Geometry check sheet. Reference: the model listing, model coordinates, mm. A direction names the side the tool comes from. Give positions to 0.01 mm unless a question says otherwise; leave off trailing zeros. Loops run counter-clockwise (first coordinate to the right, second up) from the corner with the lowest first, then second, coordinate; pieces in that order, holes last.
1. Cross-section at D-D, the plane z = 15. Record the cut outline in (x, y) (3 decimals), plus the area to 3 significant figures.
2. Release check for a two-part mould opening along Z. For faces 3 (the flat face through (29, 0, -10)), 4 (the cylindrical face through (26.91, -10.46, 0.07)), 5 (the cylindrical face through (30.15, -5.63, -12.5)) record: +Z half, -Z half, draft (parallel to the pull), parting line (faces both ways), or undercut.
3. Material ranges on L1, parallel to Z at x = 0, y = -5.75; L2, parallel to Y at x = -23, z = 17.5 (3 decimals); L3, parallel to X at y = -7.5, z = -22.5, recorded low to high.
4. Cross-section at C-C, the plane x = 0. Record the cut outline in (y, z) (3 decimals).
5. Cross-section at B-B, the plane z = 0. Record the cut outline in (x, y) (3 decimals), plus the area to 3 significant figures.
6. Tool access check on faces 1 (the cylindrical face through (-23.89, -10.46, 0.07)), 2 (the flat face through (0, -9.525, 0)). Record the directions out of +Z, -Z, +X, -X, +Y, -Y that give a thin tool (end or side, any length) a straight path to the whole face; none if there is none.
7. Cross-section at A-A, the plane x = 25.4. Record the cut outline in (y, z) (3 decimals).
8. Go/stop test with flat-tipped pins: pin 1 Ø4 at (x, z) = (-7.5, 2) entering from +Y (3 decimals); pin 2 Ø4 at (x, y) = (6.5, -9) entering from -Z; pin 3 Ø4 at (x, y) = (-24.5, -7.5) entering from +Z. Record where each tip stops, or that it passes through.
from build123d import *

# Parameters (mm, degrees)
F0_R     = 32.639
F1_DEPTH = 11.43
F2_R     = 30.353
F3_DEPTH = 9.525
F4_R     = 1.5113
F5_DEPTH = 1.905


with BuildPart() as f1:
    # F0 (on Front) → F1 (new body)
    with BuildSketch(Plane.XZ):
        Circle(F0_R)
    extrude(amount=F1_DEPTH)

    # F2 (on face) → F3 (cut)
    with BuildSketch(Plane(origin=(0, 0, 0), x_dir=(-1, 0, 0), z_dir=(0, 1, 0))):
        Circle(F2_R)
    extrude(amount=-F3_DEPTH, mode=Mode.SUBTRACT)

    # F4 (on face) → F5 (cut)
    with BuildSketch(Plane(origin=(0, -9.525, 0), x_dir=(-1, 0, 0), z_dir=(0, 1, 0))):
        with Locations((-25.4, 0)):
            Circle(F4_R)
        with Locations((25.4, 0)):
            Circle(F4_R)
    extrude(amount=-F5_DEPTH, mode=Mode.SUBTRACT)


solid = f1.part
Result:
1. outline: (-28.988, -11.43) - (28.988, -11.43) - (28.988, 0) - (26.388, 0) - (26.388, -9.525) - (-26.388, -9.525) - (-26.388, 0) - (-28.988, 0) - close
1. area: 160 mm2
2. face 3: draft
2. face 4: undercut
2. face 5: parting line
3. L1: z = -32.64 to -30.35, 30.35 to 32.64
3. L2: y = -11.43 to -9.525
3. L3: x = -23.64 to -20.37, 20.37 to 23.64
4. outline: (-11.43, -32.639) - (0, -32.639) - (0, -30.353) - (-9.525, -30.353) - (-9.525, 30.353) - (0, 30.353) - (0, 32.639) - (-11.43, 32.639) - close
5. outline: (-32.639, -11.43) - (-26.911, -11.43) - (-26.911, -9.525) - (-30.353, -9.525) - (-30.353, 0) - (-32.639, 0) - close; (-23.889, -11.43) - (23.889, -11.43) - (23.889, -9.525) - (-23.889, -9.525) - close; (26.911, -11.43) - (32.639, -11.43) - (32.639, 0) - (30.353, 0) - (30.353, -9.525) - (26.911, -9.525) - close
5. area: 156 mm2
6. face 1: +Y, -Y
6. face 2: +Y
7. outline: (-11.43, -20.497) - (0, -20.497) - (0, -16.618) - (-9.525, -16.618) - (-9.525, -1.511) - (-11.43, -1.511) - close; (-11.43, 1.511) - (-9.525, 1.511) - (-9.525, 16.618) - (0, 16.618) - (0, 20.497) - (-11.43, 20.497) - close
8. pin 1: stops at y = -9.525
8. pin 2: stops at z = -32.33
8. pin 3: stops at z = 23.64
